Geometry check sheet. Reference: the model listing, model coordinates, mm. Face numbers are marked on the shaded views. A direction names the side the tool comes from. Coordinates: 2 decimals unless noted, no trailing zeros. Write each loop counter-clockwise with the first axis right and the second up, starting at its lowest first coordinate (ties: lowest second). Pieces come first, ordered by that corner, then holes. Notation, with made-up numbers: (9.5, 31.25) -> (13.5, 31.25) arc R22 cw to (13.5, 60.25) -> close; hole circle Ø5 at (79.25, 84). An arc over 180 degrees is marked (long way). One line per question, with ' | ' between items.
```python
from build123d import *

# Parameters (mm, degrees)
SKETCH1_W                = 36.84
SKETCH1_H                = 20
BOSS_EXTRUDE1_DEPTH      = 4.7
SKETCH2_W                = 1.3
SKETCH2_H                = 2.5
BOSS_EXTRUDE2_DEPTH      = 15
BOSS_EXTRUDE2_DEPTH_BACK = 10


with BuildPart() as part:
    # Sketch1 → Boss-Extrude1 (new body)
    with BuildSketch(Plane(origin=(0, 0, 0), x_dir=(1, 0, 0), z_dir=(0, 1, 0))):
        with Locations((18.42, -10)):
            Rectangle(SKETCH1_W, SKETCH1_H)
    extrude(amount=BOSS_EXTRUDE1_DEPTH)

    # Sketch2 → Boss-Extrude2 (add, two sides)
    with BuildSketch(Plane.XY.offset(20)) as boss_extrude2_sk:
        with Locations((37.49, 2.35)):
            Rectangle(SKETCH2_W, SKETCH2_H)
    extrude(amount=BOSS_EXTRUDE2_DEPTH)
    extrude(boss_extrude2_sk.sketch, amount=-BOSS_EXTRUDE2_DEPTH_BACK)


solid = part.part
```
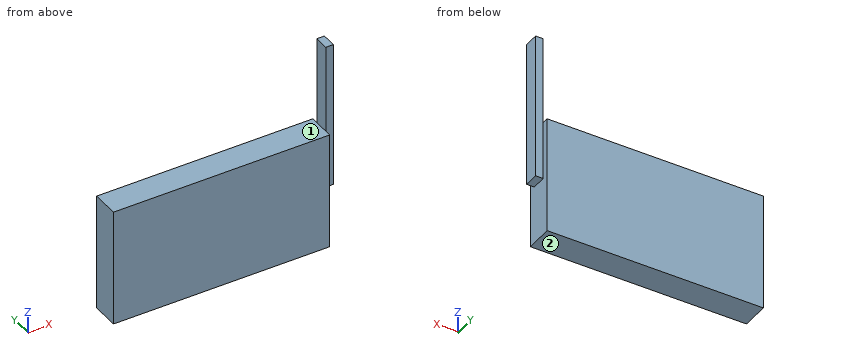
(1) Cross-section at D-D (z = 28). Record the cut outline in (x, y), plus the area to 3 significant figures.
Answers below:
outline: (36.84, 1.1) -> (38.14, 1.1) -> (38.14, 3.6) -> (36.84, 3.6) -> close | area: 3.25 mm²
(2) Cross-section at B-B (y = 2.8). Record the cut outline in (x, z), plus the area to 3 significant figures.
Answers below:
outline: (0, 0) -> (36.84, 0) -> (36.84, 10) -> (38.14, 10) -> (38.14, 35) -> (36.84, 35) -> (36.84, 20) -> (0, 20) -> close | area: 769 mm²
(3) Depth check by flat-ended pin: P1, Ø1, axis at x = 37.5, z = 24.5, coming from the +Y side; P2, Ø1.4, axis at x = 37.5, y = 2.5, coming from the -Z side; P3, Ø2.5, axis at x = 10, y = 3.5, coming from the +Z side; P4, Ø0.8, axis at y = 2, z = 28, coming from the -X side. Enter the tip coordinate at first touch or a pass-through.
Answers below:
P1: stops at y = 3.6 | P2: stops at z = 0 | P3: stops at z = 20 | P4: stops at x = 36.84
(4) Tool access check on the marked faces 1 and 2. Record the directions out of +Z, -Z, +X, -X, +Y, -Y that give a thin tool (end or side, any length) a straight path to the whole face; none if there is none.
Answers below:
face 1: +Z, -X, +Y, -Y | face 2: -Z, +X, -X, +Y, -Y
(5) Cross-section at A-A (z = 17.5). Record the cut outline in (x, y), plus the area to 3 significant figures.
Answers below:
outline: (0, 0) -> (36.84, 0) -> (36.84, 1.1) -> (38.14, 1.1) -> (38.14, 3.6) -> (36.84, 3.6) -> (36.84, 4.7) -> (0, 4.7) -> close | area: 176 mm²
(6) Material ranges on line 1 (X direction, y = 4.15, z = 2.5); line 2 (Z direction, x = 30.5, y = 3.6); line 3 (X direction, y = 2.65, z = 24), recorded low to high.
Answers below:
line 1: x = 0 to 36.84 | line 2: z = 0 to 20 | line 3: x = 36.84 to 38.14
(7) Cross-section at C-C (x = 7.5). Record the cut outline in (y, z), plus the area to 3 significant figures.
Answers below:
outline: (0, 0) -> (4.7, 0) -> (4.7, 20) -> (0, 20) -> close | area: 94.0 mm²
